Check sheet for the modelled part. Datum: model origin and axes. Units: mm. A direction names the side the tool comes from. Round coordinates to 2 decimals unless told otherwise and drop trailing zeros. Loops run counter-clockwise (first coordinate to the right, second up) from the corner with the lowest first, then second, coordinate; pieces in that order, holes last. Notation, with made-up numbers: (61, 37) -> (116, 37) arc R13 ccw to (116, 60) -> close; hole circle Ø6 at (-27.75, -7.75). An arc over 180 degrees is marked (long way). One line per item, written item: value. Start each with the question number.
1. Go/stop test with flat-tipped pins: pin 1 (8 mm diameter, centred on y = -26.5, z = 164.5, fed in from -X); pin 2 (10 mm diameter, centred on y = 8.5, z = 154.5, fed in from +X); pin 3 (2 mm diameter, centred on y = 3.5, z = 161.5, fed in from -X). Record where each tip stops, or that it passes through.
2. Cross-section at D-D on z = 149.08. Record the cut outline in (x, y), then the cut area to 3 significant figures.
3. Material ranges on L1, parallel to Z at x = 0, y = 4; L2, parallel to Y at x = -0.5, z = 164; L3, parallel to X at y = -23, z = 149, recorded low to high.
4. Release check for a two-part mould opening along X. For faces 4 (the face through (-0.846, -7.455, 155.525)), 5 (the face through (-7.262, -39.703, 167.699)), 6 (the face through (-5.1, 25.4, 164.353)) record: +X half, -X half, draft (parallel to the pull), parting line (faces both ways), or undercut.
5. Cross-section at C-C on x = 9.5. Record the cut outline in (y, z).
6. Set-up check for faces 1 (the face through (-7.045, -38.727, 151.212)), 2 (the face through (5.1, 25.4, 173.207)), 3 (the face through (5.1, 25.4, 166.58)): record each of +Z, -Z, +X, -X, +Y, -Y from which the full face is reachable in a straight line by a thin tool's end or side.
from build123d import *

# Parameters (mm, degrees)
SKETCH010_R          = 32.5
PAD005_DEPTH         = 45
SKETCH011_R          = 6.5
POCKET006_DEPTH      = 32.501
POCKET006_DEPTH_BACK = 32.501
SKETCH013_W          = 1
SKETCH013_H          = 2.20711
SKETCH013_H_2        = 2.207111


with BuildPart() as part:
    # Sketch010 → Pad005 (new body)
    with BuildSketch(Plane.XY):
        Circle(SKETCH010_R)
    extrude(amount=PAD005_DEPTH)

    # Sketch011 → Pocket006 (cut, two sides)
    with BuildSketch(Plane.XZ) as pocket006_sk:
        with Locations((0, 8.5)):
            Circle(SKETCH011_R)
    extrude(amount=-POCKET006_DEPTH, mode=Mode.SUBTRACT)
    extrude(pocket006_sk.sketch, amount=POCKET006_DEPTH_BACK, mode=Mode.SUBTRACT)

    # Sketch013 → Revolution (revolve)
    with BuildSketch(Plane.XZ):
        Polygon((32.492016, 21.565427), (33.5, 21.565427), (33.5, 23.772537), (32.487373, 23.772537), align=None)
        with Locations((33, 27.103555)):
            Rectangle(SKETCH013_W, SKETCH013_H)
        with Locations((33, 31.523173)):
            Rectangle(SKETCH013_W, SKETCH013_H_2)
    revolve(axis=Axis((0, 0, 0), (0, 0, 1)))


with BuildPart() as part_1:
    # Body003 placement: moved
    add(part.part.moved(Location((0, -7, 140.58))))


solid = part_1.part
Taken from the geometry:
1. pin 1: stops at x = -29.7
1. pin 2: stops at x = 30.76
1. pin 3: stops at x = -32.05
2. outline: (-6.5, -38.84) -> (-6.5, 24.84) arc R32.5 ccw to start; (6.5, -38.84) arc R32.5 ccw to (6.5, 24.84) -> close
2. area: 2,480 mm2
3. L1: z = 140.58 to 142.58, 155.58 to 185.58
3. L2: y = -40.5 to 26.5
3. L3: x = -28.29 to -6.5, 6.5 to 28.29
4. face 4: undercut
4. face 5: parting line
4. face 6: draft
5. outline: (-39.12, 162.15) -> (-38.08, 162.15) -> (-38.08, 140.58) -> (24.08, 140.58) -> (24.08, 162.15) -> (25.12, 162.15) -> (25.12, 164.35) -> (24.08, 164.35) -> (24.08, 166.58) -> (25.12, 166.58) -> (25.12, 168.79) -> (24.08, 168.79) -> (24.08, 171) -> (25.12, 171) -> (25.12, 173.21) -> (24.08, 173.21) -> (24.08, 185.58) -> (-38.08, 185.58) -> (-38.08, 173.21) -> (-39.12, 173.21) -> (-39.12, 171) -> (-38.08, 171) -> (-38.08, 168.79) -> (-39.12, 168.79) -> (-39.12, 166.58) -> (-38.08, 166.58) -> (-38.08, 164.35) -> (-39.12, 164.35) -> close
6. face 1: -Z
6. face 2: +Z
6. face 3: none
